Check sheet for the modelled part. Datum: model origin and axes. Units: mm. Give positions to 0.01 mm unless a question says otherwise; leave off trailing zeros. Order: outer loops, then holes, each group sorted by start corner. A loop starts at its lowest first (then second) coordinate and runs counter-clockwise, first axis right, second up. Notation, with made-up numbers: (8, -26.5) -> (64, -26.5) arc R6 ccw to (64, -21.5) -> close; hole circle Ø2 at (10.25, -36). An arc over 180 degrees is marked (long way). One line per question, with ' | ' between items.
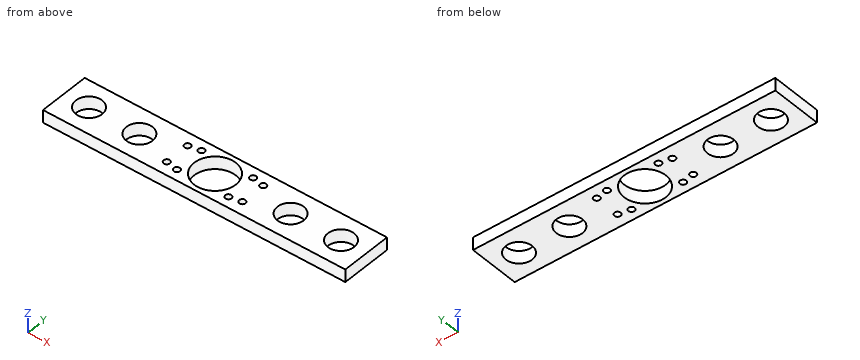
Autodesk Inventor part; units mm, degrees
ref_plane "Work Plane1" through (-30.9265, 0, 3.175) normal (0, -1, 0) x (1, 0, 0)
ref_plane "Work Plane2" through (0, 12.6269, 3.175) normal (-1, 0, 0) x (0, -1, 0)
ref_plane "YZ Plane" through (0, 0, 0) normal (1, 0, 0) x (0, 1, 0)
sketch "Sketch1" plane through (0, 0, 0) normal (0, 0, 1) x (1, 0, 0)
  circle A0 centre (0, 0) radius 6.477 construction
  circle A1 centre (0, 0) radius 4.75 construction
  circle A2 centre (0, 0) radius 9.525 construction
  line L0 (-38.1, -6.35) -> (38.1, -6.35) construction
  line L1 (38.1, -6.35) -> (38.1, 6.35) construction
  line L2 (38.1, 6.35) -> (-38.1, 6.35) construction
  line L3 (-38.1, 6.35) -> (-38.1, -6.35) construction
  line L4 (-38.1, 6.35) -> (38.1, 6.35)
  line L5 (38.1, 6.35) -> (38.1, -6.35)
  line L6 (38.1, -6.35) -> (-38.1, -6.35)
  line L7 (-38.1, -6.35) -> (-38.1, 6.35)
  dimension "d0" = 12.954
  dimension "d1" = 9.5
  dimension "d2" = 19.05
  dimension "d3" = 76.2
  dimension "d4" = 12.7
extrude "Extrusion1" add sketch "Sketch1" along normal blind 3.175
sketch "Sketch2" plane through (0, 0, 3.175) normal (0, 0, 1) x (1, 0, 0)
  circle A0 centre (0, 0) radius 5.25
  dimension "d7" = 10.5
extrude "Extrusion2" cut sketch "Sketch2" against normal through all
sketch "Sketch4" plane through (0, 0, 3.175) normal (0, 0, 1) x (1, 0, 0)
  circle A0 centre (0, 0) radius 5.25
  circle A1 centre (0, 0) radius 7.5 construction
  arc A2 (6.4952, 3.75) -> (-6.4952, 3.75) centre (0, 0) ccw construction
  line L0 (0, 0) -> (6.4952, 3.75) construction
  line L1 (0, 0) -> (7.5, 0) construction
  line L2 (0, 0) -> (-6.4952, 3.75) construction
  point P0 (6.4952, 3.75)
  dimension "d13" = 15
  dimension "d14" = 30
  dimension "d15" = 120
hole "Hole1" at (-6.4952, 3.75, 3.175) at (6.4952, 3.75, 3.175) direction (0, 0, -1) diameter 1.5748 end through all
sketch "Sketch5" plane through (0, 0, 3.175) normal (0, 0, 1) x (1, 0, 0)
  circle A0 centre (6.4952, 3.75) radius 0.7874
  circle A1 centre (-6.4952, 3.75) radius 0.7874
  circle A2 centre (0, 0) radius 5.25
  line L0 (38.1, -6.35) -> (-38.1, -6.35)
  line L1 (38.1, 6.35) -> (38.1, -6.35)
  line L2 (-38.1, 6.35) -> (38.1, 6.35)
  line L3 (-38.1, -6.35) -> (-38.1, 6.35)
  line L4 (-30.9265, 0) -> (29.6642, 0) construction
ref_plane "Work Plane1" through (-30.9265, 0, 3.175) normal (0, -1, 0) x (1, 0, 0)
mirror "Mirror1" about plane through (-30.9265, 0, 3.175) normal (0, -1, 0) of "Hole1"
sketch "Sketch6" plane through (0, 0, 3.175) normal (0, 0, 1) x (1, 0, 0)
  point P0 (-31.75, 0)
  point P1 (-19.05, 0)
hole "Hole2" at (-31.75, 0, 3.175) at (-19.05, 0, 3.175) direction (0, 0, -1) diameter 6.604 end through all
sketch "Sketch7" plane through (0, 0, 3.175) normal (0, 0, 1) x (1, 0, 0)
  circle A0 centre (-19.05, 0) radius 3.302
  circle A1 centre (-31.75, 0) radius 3.302
  circle A2 centre (6.4952, -3.75) radius 0.7874
  circle A3 centre (-6.4952, -3.75) radius 0.7874
  circle A4 centre (6.4952, 3.75) radius 0.7874
  circle A5 centre (-6.4952, 3.75) radius 0.7874
  circle A6 centre (0, 0) radius 5.25
  line L0 (38.1, -6.35) -> (-38.1, -6.35)
  line L1 (38.1, 6.35) -> (38.1, -6.35)
  line L2 (-38.1, 6.35) -> (38.1, 6.35)
  line L3 (-38.1, -6.35) -> (-38.1, 6.35)
  line L4 (0, 12.6269) -> (0, -12.6269) construction
ref_plane "Work Plane2" through (0, 12.6269, 3.175) normal (-1, 0, 0) x (0, -1, 0)
mirror "Mirror2" about plane through (0, 12.6269, 3.175) normal (-1, 0, 0) of "Hole2"
sketch "Sketch8" plane through (0, 0, 3.175) normal (0, 0, 1) x (1, 0, 0)
  point P0 (-9.525, -3.175)
  point P1 (-9.525, 3.175)
  point P2 (9.525, 3.175)
  point P3 (9.525, -3.175)
hole "Hole3" at (-9.525, 3.175, 3.175) at (-9.525, -3.175, 3.175) at (9.525, -3.175, 3.175) at (9.525, 3.175, 3.175) direction (0, 0, -1) diameter 1.5748 end through all
properties part number "simple_chuck"
Q1. Thickness scan on line 1 (Y direction, x = -6, z = 0.7); line 2 (X direction, y = -2, z = 1.95); line 3 (X direction, y = -1, z = 1.45). Record the ranges inside material, lowest first.
Result sheet:
line 1: y = -6.35 to -4.36, -3.14 to 3.14, 4.36 to 6.35 | line 2: x = -38.1 to -34.38, -29.12 to -21.68, -16.42 to -4.85, 4.85 to 16.42, 21.68 to 29.12, 34.38 to 38.1 | line 3: x = -38.1 to -34.9, -28.6 to -22.2, -15.9 to -5.15, 5.15 to 15.9, 22.2 to 28.6, 34.9 to 38.1
Q2. Section check C-C (z = 1.75). Count the separate pieces of the cut face and the enclosed holes in it, and give its area (3 significant figures).
Result sheet:
separate pieces: 1 | enclosed holes: 13 | area: 729 mm2
Q3. Section check B-B (y = 0). Enter the section's corners in (x, z) (3 decimals).
Result sheet:
outline: (-38.1, 0) -> (-35.052, 0) -> (-35.052, 3.175) -> (-38.1, 3.175) -> close; (-28.448, 0) -> (-22.352, 0) -> (-22.352, 3.175) -> (-28.448, 3.175) -> close; (-15.748, 0) -> (-5.25, 0) -> (-5.25, 3.175) -> (-15.748, 3.175) -> close; (5.25, 0) -> (15.748, 0) -> (15.748, 3.175) -> (5.25, 3.175) -> close; (22.352, 0) -> (28.448, 0) -> (28.448, 3.175) -> (22.352, 3.175) -> close; (35.052, 0) -> (38.1, 0) -> (38.1, 3.175) -> (35.052, 3.175) -> close
Q4. Section check A-A (x = -31.75). Enter the section's corners in (y, z) (3 decimals), and give its area (3 significant figures).
Result sheet:
outline: (-6.35, 0) -> (-3.302, 0) -> (-3.302, 3.175) -> (-6.35, 3.175) -> close; (3.302, 0) -> (6.35, 0) -> (6.35, 3.175) -> (3.302, 3.175) -> close | area: 19.4 mm2
Q5. Depth check by flat-ended pin: pin 1 Ø6 at (x, y) = (-31.75, 0) entering from +Z. Enter the tip coordinate at first touch or a pass-through.
Result sheet:
pin 1: passes through
Q6. Section check D-D (x = 0). Enter the section's corners in (y, z) (3 decimals), and give its area (4 significant figures).
Result sheet:
outline: (-6.35, 0) -> (-5.25, 0) -> (-5.25, 3.175) -> (-6.35, 3.175) -> close; (5.25, 0) -> (6.35, 0) -> (6.35, 3.175) -> (5.25, 3.175) -> close | area: 6.985 mm2
